from build123d import *

# Parameters (mm, degrees)
BOSS_EXTRUDE1_DEPTH = 5
FILLET1_R           = 1


with BuildPart() as part:
    # Sketch1 → Boss-Extrude1 (new body)
    with BuildSketch(Plane.XY):
        Polygon((29.405194241, 5), (46.088102842, 5), (46.088102842, 0), (226.188102842, 0), (226.188102842, 5), (246.060241867, 5), (222.607000141, 11.097188159), (221.348957412, 6.258042728), (134.244339671, 28.902811841), (135.5023824, 33.741957272), (130.044499116, 35.16085457), (124.405194241, 35.16085457), (124.405194241, 30.16085457), (34.405194241, 30.16085457), (34.405194241, 35.16085457), (29.405194241, 35.16085457), align=None)
    extrude(amount=BOSS_EXTRUDE1_DEPTH)

    # Fillet1
    fillet1_edges = [part.edges().sort_by_distance(p)[0] for p in [
        (130.044499116, 35.16085457, 2.5),
        (135.5023824, 33.741957272, 2.5),
        (222.607000141, 11.097188159, 2.5),
        (226.188102842, 0, 2.5),
        (46.088102842, 0, 2.5),
        (34.405194241, 35.16085457, 2.5),
        (124.405194241, 35.16085457, 2.5),
    ]]
    fillet(fillet1_edges, radius=FILLET1_R)


solid = part.part
For this review, take the finished solid that the model builds, in its own axes (mm). A direction names the side the tool comes from. Round coordinates to 2 decimals unless told otherwise and drop trailing zeros. Order: outer loops, then holes, each group sorted by start corner. A loop starts at its lowest first (then second) coordinate and runs counter-clockwise, first axis right, second up. Notation, with made-up numbers: M 51,-39.75 L 71,-39.75 A18 ccw 71,-9.75 Z; hole C -23,-21 d2. An arc over 180 degrees is marked long. Write each question's results on one line, items separated by ' | '. Start each with the question number.
1. Add section C-C (y = 15). State the section outline as (x, z) points, then the cut area to 3 significant figures.
2. To check wall thickness, follow L1, parallel to Y at x = 75.5, z = 0.95; L2, parallel to X at y = 30, z = 1.7; L3, parallel to Y at x = 44.5, z = 1.65. State the ranges of each line that lie inside material, in increasing order. Write a range as [from, to].
3. Draft analysis for pull direction Y (two halves, no side actions). For faces 4 (the face through (221.86, 8.22, 2.46)), 5 (the face through (124.405, 32, 2)), 6 (the face through (134.74, 30.81, 2.46)), state which applies: pulls with the +Y half, pulls with the -Y half, needs draft (parallel to the pull), parting line crosses it, or undercut.
4. Clearance check with flat-ended pins moving along their axes: pin 1 Ø3 at (x, y) = (79.5, 8.5) entering from -Z; pin 2 Ø1.5 at (x, z) = (84, 2) entering from +Y; pin 3 Ø2.5 at (x, z) = (39, 1.5) entering from -Y; pin 4 Ø3 at (x, y) = (139, 30.5) entering from -Z. State where each tip first meets the part, or that it passes through.
5. Add section B-B (x = 80.5). State the section outline as (y, z) points.
6. Tool access review of faces 1 (the face through (226.188, 3, 2)), 2 (the face through (34.405, 32, 2)), 3 (the face through (46.088, 3, 2)): name each direction out of +Z, -Z, +X, -X, +Y, -Y from which nothing blocks a thin tool from reaching the whole face with its end or side.
7. Add section A-A (z = 2.15). State the section outline as (x, y) points, then the cut area to 3 significant figures.
Output values:
1) outline: M 29.41,0 L 187.72,0 L 187.72,5 L 29.41,5 Z | area: 792 mm^2
2) L1: [0, 30.16] | L2: [29.41, 134.53] | L3: [5, 30.16]
3) face 4: pulls with the +Y half | face 5: needs draft | face 6: undercut
4) pin 1: z = 0 | pin 2: y = 30.16 | pin 3: y = 5 | pin 4: through
5) outline: M 0,0 L 30.16,0 L 30.16,5 L 0,5 Z
6) face 1: +Z, -Z, +X, -Y | face 2: +Z, -Z, +Y | face 3: +Z, -Z, -X, -Y
7) outline: M 29.41,5 L 46.09,5 L 46.09,1 A1 ccw 47.09,0 L 225.19,0 A1 ccw 226.19,1 L 226.19,5 L 246.06,5 L 223.57,10.85 A1 ccw 222.36,10.13 L 221.35,6.26 L 134.24,28.9 L 135.25,32.77 A1 ccw 134.53,33.99 L 130.17,35.13 A1 ccw 129.92,35.16 L 125.41,35.16 A1 ccw 124.41,34.16 L 124.41,30.16 L 34.41,30.16 L 34.41,34.16 A1 ccw 33.41,35.16 L 29.41,35.16 Z | area: 4,780 mm^2
